Part print with two shaded views. Sizes in mm from the minimum x, y, z corner. A direction names the side the tool comes from. Give positions to 0.01 mm unless a question says otherwise; leave off trailing zeros. Order: outer loops, then holes, each group sorted by start corner. A loop starts at its lowest first (then second) coordinate and runs counter-clockwise, first axis right, second up. Notation, with made-up numbers: (47.5, 75.25) -> (102.5, 75.25) arc R16 cw to (102.5, 93.25) -> close; hole circle Ø1 at (-8, -7.5). An arc over 180 degrees is marked (long way). Write item = value, one per line. Start each with the question number.
Item 1: Band-saw the part on A-A on z = 15.5. Write the cut outline in (x, y) (1 decimal).
Item 2: Drill centre lines: line 1 along X through (y, z) = (43.5, 23) (1 decimal); line 2 along Y through (x, z) = (64, 25); line 3 along Z through (x, y) = (30, 51.5). Where is each one in solid material? Low to high.
Item 3: Tool access for the marked faces 1 and 2: list every direction of +Z, -Z, +X, -X, +Y, -Y with a clear straight run to the whole face (end or side of a thin tool).
Item 4: Band-saw the part on B-B on y = 35. Write the cut outline in (x, z) (1 decimal).
Item 5: Pull direction X, two halves, no side cores. Call the marked faces 3, 4 and 5: +X half, -X half, draft (parallel to the pull), parting line (faces both ways), or undercut.
Item 6: Flat gauge pin, fed straight in: P1, Ø13.5, axis at x = 36, y = 43, coming from the +Z side. Where does the tip first touch, or does it go through?
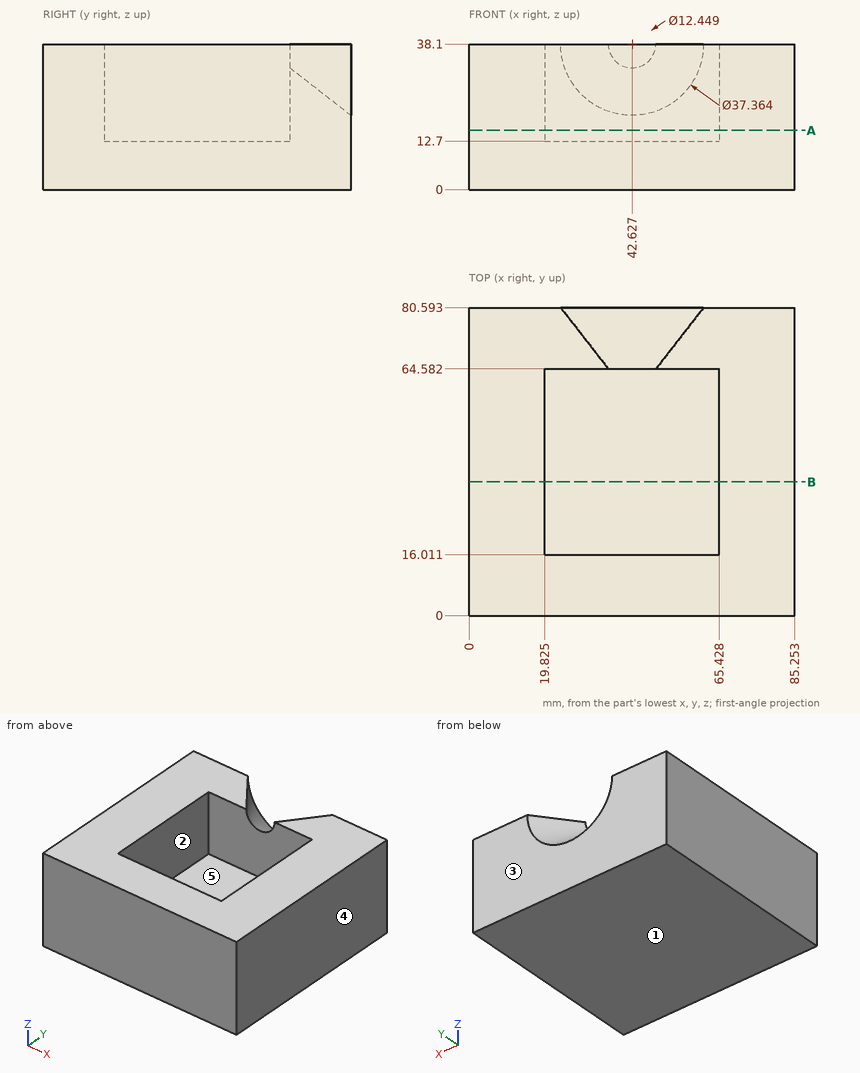
Values found:
q1.outline = (0, 0) -> (85.3, 0) -> (85.3, 80.6) -> (0, 80.6) -> close; hole (19.8, 16) -> (65.4, 16) -> (65.4, 64.6) -> (19.8, 64.6) -> close
q2.line_1 = 0 to 19.8, 65.4 to 85.3
q2.line_2 = 0 to 16.01, 64.58 to 80.59
q2.line_3 = 0 to 12.7
q3.face_1 = -Z, +X, -X, +Y, -Y
q3.face_2 = +Z
q4.outline = (0, 0) -> (85.3, 0) -> (85.3, 38.1) -> (65.4, 38.1) -> (65.4, 12.7) -> (19.8, 12.7) -> (19.8, 38.1) -> (0, 38.1) -> close
q5.face_3 = draft
q5.face_4 = +X half
q5.face_5 = undercut
q6.P1 = 12.7
